Check sheet for the modelled part. Datum: model origin and axes. Units: mm. Round coordinates to 2 decimals unless told otherwise and drop trailing zeros. Loops run counter-clockwise (first coordinate to the right, second up) from the corner with the lowest first, then second, coordinate; pieces in that order, holes last. Notation, with made-up numbers: (36, -10.75) - (63, -10.75) arc R17 cw to (63, 13.25) - close; hole circle Ø1 at (69.25, 44). An arc over 180 degrees is marked (long way). Answer in a Markdown table with one row per item. Add a question column.
(1) Cross-section at A-A on x = 0. Enter the section's corners in (y, z), then the cut area to 4 significant figures.
(2) Cross-section at C-C on y = 24. Enter the section's corners in (x, z).
(3) Mould release check, pull along Y, two halves, no side actions. Record for faces 1 (the cylindrical face through (0.923, 150.726, 1.479)), 2 (the flat face through (-5, 77, 1)), 3 (the cylindrical face through (0.1, 157.5, 1.5)): +Y half, -Y half, draft (parallel to the pull), parting line (faces both ways), or undercut.
(4) Thickness scan on line 1 along Y through (x, z) = (0, 1.3); line 2 along Y through (x, z) = (-1.5, 2.25); line 3 along Y through (x, z) = (-2.75, 1.85). Record the ranges inside material, lowest first.
(5) Gauge pin test, flat end, axial feed: pin 1 (3.5 mm diameter, centred on x = 0, y = 24, fed in from -Z). Record the tip position at first contact, or that the pin passes through.
(6) Cross-section at B-B on z = 1.55. Enter the section's corners in (x, y).
from build123d import *

# Parameters (mm, degrees)
SKETCH1_R           = 2
SKETCH1_R_2         = 5
BOSS_EXTRUDE1_DEPTH = 3


with BuildPart() as part:
    # Sketch1 → Boss-Extrude1 (new body)
    # profile 1 of 3: a face of its own
    with BuildSketch(Plane.XY):
        with BuildLine():
            Line((-5, 152.5), (-5, 0))
            ThreePointArc((-5, 0), (0, 5), (5, 0))
            Line((5, 0), (5, 152.5))
            ThreePointArc((5, 152.5), (0, 147.5), (-5, 152.5))
        make_face()
        with Locations((0, 24)):
            Circle(SKETCH1_R, mode=Mode.SUBTRACT)
    # profile 2 of 3: a face of its own
    with BuildSketch(Plane.XY):
        with Locations((0, 152.5)):
            Circle(SKETCH1_R_2)
        with Locations((0, 152.5)):
            Circle(SKETCH1_R, mode=Mode.SUBTRACT)
    # profile 3 of 3: a face of its own
    with BuildSketch(Plane.XY):
        Circle(SKETCH1_R_2)
        Circle(SKETCH1_R, mode=Mode.SUBTRACT)
    extrude(amount=BOSS_EXTRUDE1_DEPTH)


solid = part.part
Answers:
| question | item | result |
|---|---|---|
| 1 | outline | (-5, 0) - (-2, 0) - (-2, 3) - (-5, 3) - close; (2, 0) - (22, 0) - (22, 3) - (2, 3) - close; (26, 0) - (150.5, 0) - (150.5, 3) - (26, 3) - close; (154.5, 0) - (157.5, 0) - (157.5, 3) - (154.5, 3) - close |
| 1 | area | 451.5 mm^2 |
| 2 | outline | (-5, 0) - (-2, 0) - (-2, 3) - (-5, 3) - close; (2, 0) - (5, 0) - (5, 3) - (2, 3) - close |
| 3 | face 1 | undercut |
| 3 | face 2 | draft |
| 3 | face 3 | +Y half |
| 4 | line 1 | y = -5 to -2, 2 to 22, 26 to 150.5, 154.5 to 157.5 |
| 4 | line 2 | y = -4.77 to -1.32, 1.32 to 22.68, 25.32 to 151.18, 153.82 to 157.27 |
| 4 | line 3 | y = -4.18 to 156.68 |
| 5 | pin 1 | passes through |
| 6 | outline | (-5, 0) arc R5 ccw to (5, 0) - (5, 152.5) arc R5 ccw to (-5, 152.5) - close; hole circle Ø4 at (0, 0); hole circle Ø4 at (0, 24); hole circle Ø4 at (0, 152.5) |
